Model file for the job. Use its own axes, mm. A direction names the side the tool comes from. Round coordinates to 2 decimals unless told otherwise and drop trailing zeros. Write each loop counter-clockwise with the first axis right and the second up, starting at its lowest first coordinate (ties: lowest second). Pieces come first, ordered by that corner, then holes. Notation, with made-up numbers: (30.25, 46) - (55.25, 46) arc R10 cw to (55.25, 62) - close; hole circle Ø6 at (1, -12). An arc over 180 degrees is marked (long way). One line per item, written item: value.
from build123d import *

# Parameters (mm, degrees)
PAD_DEPTH       = 50
SKETCH001_R     = 23.31
POCKET_DEPTH    = 7
SKETCH002_R     = 2
POCKET001_DEPTH = 7
PAD001_DEPTH    = 10


with BuildPart() as part:
    # Sketch → Pad (new body)
    with BuildSketch(Plane.XZ):
        Polygon((-41.7, -27), (-48.7, -27), (-48.7, 20), (0, 20), (0, 13), (-41.7, 13), align=None)
    extrude(amount=-PAD_DEPTH)

    # Sketch001 → Pocket (cut)
    with BuildSketch(Plane(origin=(0, 0, 20), x_dir=(-1, 0, 0), z_dir=(0, 0, 1))):
        with Locations((-8.31, -25)):
            Circle(SKETCH001_R)
    extrude(amount=-POCKET_DEPTH, mode=Mode.SUBTRACT)

    # Sketch002 → Pocket001 (cut)
    with BuildSketch(Plane(origin=(-48.7, 0, 0), x_dir=(0, 0, -1), z_dir=(-1, 0, 0))):
        with Locations((20, -25)):
            Circle(SKETCH002_R)
    extrude(amount=-POCKET001_DEPTH, mode=Mode.SUBTRACT)

    # Sketch003 → Pad001 (new body)
    with BuildSketch(Plane.XZ):
        Polygon((-41.7, 13), (-41.7, 3), (-31.7, 13), align=None)
    extrude(amount=-PAD001_DEPTH)


solid = part.part
1. Drop flat-ended pins along their axis: pin 1 (12.5 mm diameter, centred on x = -29, y = 21.5, fed in from -Z); pin 2 (5 mm diameter, centred on x = -36, z = 6, fed in from +Y); pin 3 (6 mm diameter, centred on y = 14.5, z = 13, fed in from +X). Give the stop position or say it passes through.
Report:
pin 1: z = 13
pin 2: y = 10
pin 3: x = -10.69
2. Tool access for faces 1 (the face through (-41.7, 25, -7)), 2 (the face through (-30, 25, 20)): list every direction of +Z, -Z, +X, -X, +Y, -Y with a clear straight run to the whole face (end or side of a thin tool).
Report:
face 1: -Z, +X, +Y
face 2: +Z, +X, -X, +Y, -Y
3. Band-saw the part on D-D on z = 5. Write the cut outline in (x, y).
Report:
outline: (-48.7, 0) - (-39.7, 0) - (-39.7, 10) - (-41.7, 10) - (-41.7, 50) - (-48.7, 50) - close
4. Mould opens along Y. For faces 3 (the face through (-35, 50, 14)), 4 (the face through (-37, 0, 9)), 5 (the face through (-45.2, 26.2, -18.4)), 6 (the face through (-25, 25, 13)) say: released by +Y, released by -Y, zero draft, split by the parting line, or undercut.
Report:
face 3: released by +Y
face 4: released by -Y
face 5: undercut
face 6: zero draft
5. Band-saw the part on A-A on y = 25. Write the cut outline in (x, z).
Report:
outline: (-48.7, -27) - (-41.7, -27) - (-41.7, -22) - (-48.7, -22) - close; (-48.7, -18) - (-41.7, -18) - (-41.7, 13) - (-15, 13) - (-15, 20) - (-48.7, 20) - close
6. Band-saw the part on C-C on x = -9.5. Write the cut outline in (y, z).
Report:
outline: (0, 13) - (9.96, 13) - (9.96, 20) - (0, 20) - close; (40.04, 13) - (50, 13) - (50, 20) - (40.04, 20) - close
7. Band-saw the part on B-B on z = -20. Write the cut outline in (x, y).
Report:
outline: (-48.7, 0) - (-41.7, 0) - (-41.7, 23) - (-48.7, 23) - close; (-48.7, 27) - (-41.7, 27) - (-41.7, 50) - (-48.7, 50) - close
8. Wall check: probe 1 along Z at (x, y) = (-44.5, 25); probe 2 along Y at (x, z) = (-46, -20); probe 3 along X at (y, z) = (15.5, 9). Give the ranges that are in metal, low to high. Write a range as [from, to].
Report:
probe 1: [-27, -22], [-18, 20]
probe 2: [0, 23], [27, 50]
probe 3: [-48.7, -41.7]
